Design review of the part built by this model. Coordinates are the model's own, in mm. Face numbers are marked on the shaded views. A direction names the side the tool comes from. Coordinates: 2 decimals unless noted, no trailing zeros. Loops run counter-clockwise (first coordinate to the right, second up) from the corner with the lowest first, then second, coordinate; pieces in that order, holes last.
Q1. For P1, Ø3.5, axis at x = -102, z = -38, coming from the -Y side; P2, Ø9.5, axis at x = -16.5, z = -47, coming from the -Y side; P3, Ø1.4, axis at y = -5.5, z = 9.5, coming from the -X side, all flat-tipped, find the tip position at first contact; note any pin that passes through.
Q2. Add section C-C on x = -10. Give the boundary of the cut face in (y, z).
Q3. Machinability: for the marked faces 5, 6, 7 and 8, which of the approach directions +Z, -Z, +X, -X, +Y, -Y give a long, thin tool a straight path to every point of the face, cutting with its end or side? Answer none if there is none.
Q4. Add section D-D on y = 5.75. Give the boundary of the cut face in (x, z).
Q5. Wall thickness on probe 1 along Z at (x, y) = (-45.5, -2); probe 2 along Z at (x, y) = (-34.5, -9.25); probe 3 along Z at (x, y) = (-30.5, 6): over which ranges is each line inside the solid? List them lowest first.
Q6. Add section A-A on y = 11. Give the boundary of the cut face in (x, z).
Q7. Draft analysis for pull direction X (two halves, no side actions). For the marked faces 1, 2, 3 and 4, state which applies: released by +X, released by -X, zero draft, split by the parting line, or undercut.
Q8. Add section B-B on x = -72. Give the boundary of the cut face in (y, z).
```python
from build123d import *

# Parameters (mm, degrees)
F1_DEPTH      = 14.224
F2_DEPTH      = 7.874
F3_DEPTH      = 12.7
F0_W          = 7.468818
F0_H          = 25.4
F4_DEPTH      = 3.048
F4_DEPTH_BACK = 7.874


with BuildPart() as f1:
    # F0 (on Front) → F1 (new body, symmetric)
    with BuildSketch(Plane.XZ):
        Polygon((-31.242, -14.224), (-31.242, 0), (-97.179182, 0), (-104.648, 0), (-104.648, -14.224), align=None)
    extrude(amount=F1_DEPTH, both=True)

    # F0 (on Front) → F2 (join, symmetric)
    with BuildSketch(Plane.XZ):
        Polygon((-31.242, 0), (-25.4, 0), (-11.728174, 13.671826), (-35.052, 13.671826), (-35.052, 25.4), (-75.822987, 25.4), (-97.179182, 25.4), (-97.179182, 0), align=None)
        with BuildLine():
            ThreePointArc((-75.822987, 8.69926), (-81.410987, 14.28726), (-75.822987, 19.87526))
            Line((-75.822987, 19.87526), (-41.718637, 19.87526))
            ThreePointArc((-41.718637, 19.87526), (-36.130637, 14.28726), (-41.718637, 8.69926))
            Line((-41.718637, 8.69926), (-75.822987, 8.69926))
        make_face(mode=Mode.SUBTRACT)
    extrude(amount=F2_DEPTH, both=True)

    # F0 (on Front) → F3 (join, symmetric)
    with BuildSketch(Plane.XZ):
        Polygon((-35.052, 13.671826), (-11.728174, 13.671826), (0, 25.4), (-35.052, 25.4), align=None)
    extrude(amount=F3_DEPTH, both=True)

    # F0 (on Front) → F4 (join, two sides)
    with BuildSketch(Plane.XZ) as f4_sk:
        with Locations((-100.913591, 12.7)):
            Rectangle(F0_W, F0_H)
    extrude(amount=F4_DEPTH)
    extrude(f4_sk.sketch, amount=-F4_DEPTH_BACK)

    # F5: F1 across face


with BuildPart() as f1_1:
    add(f1.part)
    add(f1.part.mirror(Plane(origin=(-67.945, 0, -14.224), x_dir=(1, 0, 0), z_dir=(0, 0, -1))))


solid = f1_1.part
```
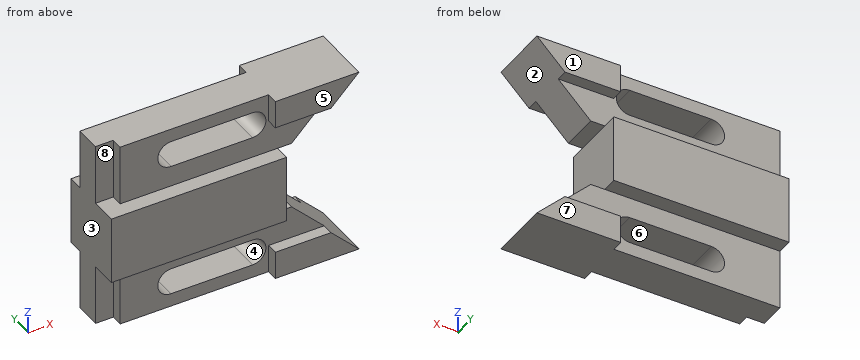
Entries:
1. P1: stops at y = -3.05
1. P2: stops at y = -12.7
1. P3: stops at x = -97.18
2. outline: (-12.7, -53.85) - (12.7, -53.85) - (12.7, -43.85) - (-12.7, -43.85) - close; (-12.7, 15.4) - (12.7, 15.4) - (12.7, 25.4) - (-12.7, 25.4) - close
3. face 5: +Z, +X, -X, -Y
3. face 6: +Y, -Y
3. face 7: -Z, +X, -X, +Y
3. face 8: +Z, -X, -Y
4. outline: (-104.65, -53.85) - (0, -53.85) - (-25.4, -28.45) - (-31.24, -28.45) - (-31.24, 0) - (-25.4, 0) - (0, 25.4) - (-104.65, 25.4) - close; hole (-75.82, -48.32) - (-41.72, -48.32) arc R5.59 ccw to (-41.72, -37.15) - (-75.82, -37.15) arc R5.59 ccw to start; hole (-75.82, 8.7) - (-41.72, 8.7) arc R5.59 ccw to (-41.72, 19.88) - (-75.82, 19.88) arc R5.59 ccw to start
5. probe 1: z = -53.85 to -48.32, -37.15 to 8.7, 19.88 to 25.4
5. probe 2: z = -53.85 to -42.12, -28.45 to 0, 13.67 to 25.4
5. probe 3: z = -53.85 to -28.45, 0 to 25.4
6. outline: (-104.65, -28.45) - (-31.24, -28.45) - (-31.24, 0) - (-104.65, 0) - close; (-35.05, -53.85) - (0, -53.85) - (-11.73, -42.12) - (-35.05, -42.12) - close; (-35.05, 13.67) - (-11.73, 13.67) - (0, 25.4) - (-35.05, 25.4) - close
7. face 1: zero draft
7. face 2: released by +X
7. face 3: released by -X
7. face 4: undercut
8. outline: (-14.22, -28.45) - (-7.87, -28.45) - (-7.87, -37.15) - (7.87, -37.15) - (7.87, -28.45) - (14.22, -28.45) - (14.22, 0) - (7.87, 0) - (7.87, 8.7) - (-7.87, 8.7) - (-7.87, 0) - (-14.22, 0) - close; (-7.87, -53.85) - (7.87, -53.85) - (7.87, -48.32) - (-7.87, -48.32) - close; (-7.87, 19.88) - (7.87, 19.88) - (7.87, 25.4) - (-7.87, 25.4) - close
